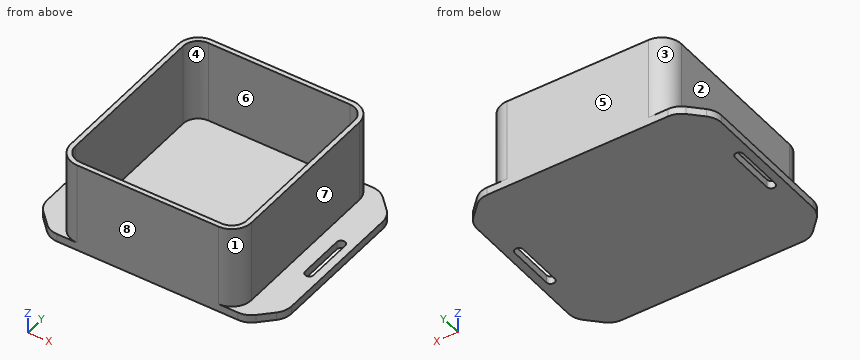
```python
from build123d import *

# Parameters (mm, degrees)
F1_DEPTH = 2
F3_DEPTH = 21


with BuildPart() as f1:
    # F0 (on Top) → F1 (new body)
    with BuildSketch(Plane.XY):
        with BuildLine():
            Line((-60.535534, 4.535534), (-57.464466, 1.464466))
            ThreePointArc((-57.464466, 1.464466), (-55.842349, 0.380602), (-53.928932, 0))
            Line((-53.928932, 0), (-8.071068, 0))
            ThreePointArc((-8.071068, 0), (-6.157651, 0.380602), (-4.535534, 1.464466))
            Line((-4.535534, 1.464466), (-1.464466, 4.535534))
            ThreePointArc((-1.464466, 4.535534), (-0.380602, 6.157651), (0, 8.071068))
            Line((0, 8.071068), (0, 41.928932))
            ThreePointArc((0, 41.928932), (-0.380602, 43.842349), (-1.464466, 45.464466))
            Line((-1.464466, 45.464466), (-4.535534, 48.535534))
            ThreePointArc((-4.535534, 48.535534), (-6.157651, 49.619398), (-8.071068, 50))
            Line((-8.071068, 50), (-53.928932, 50))
            ThreePointArc((-53.928932, 50), (-55.842349, 49.619398), (-57.464466, 48.535534))
            Line((-57.464466, 48.535534), (-60.535534, 45.464466))
            ThreePointArc((-60.535534, 45.464466), (-61.619398, 43.842349), (-62, 41.928932))
            Line((-62, 41.928932), (-62, 8.071068))
            ThreePointArc((-62, 8.071068), (-61.619398, 6.157651), (-60.535534, 4.535534))
        make_face()
        with BuildLine():
            Line((-60, 19.118238), (-60, 30.881762))
            ThreePointArc((-60, 30.881762), (-58.930589, 31.951173), (-57.861177, 30.881762))
            Line((-57.861177, 30.881762), (-57.861177, 19.118238))
            ThreePointArc((-57.861177, 19.118238), (-58.930589, 18.048827), (-60, 19.118238))
        make_face(mode=Mode.SUBTRACT)
        with BuildLine():
            Line((-4.138823, 19.118238), (-4.138823, 30.881762))
            ThreePointArc((-4.138823, 30.881762), (-3.069411, 31.951173), (-2, 30.881762))
            Line((-2, 30.881762), (-2, 19.118238))
            ThreePointArc((-2, 19.118238), (-3.069411, 18.048827), (-4.138823, 19.118238))
        make_face(mode=Mode.SUBTRACT)
    extrude(amount=F1_DEPTH)

    # F2 (on face) → F3 (join)
    with BuildSketch(Plane.XY.offset(2)):
        with BuildLine():
            ThreePointArc((-13.071068, 0), (-9.535534, 1.464466), (-8.071068, 5))
            Line((-8.071068, 5), (-8.071068, 45))
            ThreePointArc((-8.071068, 45), (-9.535534, 48.535534), (-13.071068, 50))
            Line((-13.071068, 50), (-48.928932, 50))
            ThreePointArc((-48.928932, 50), (-52.464466, 48.535534), (-53.928932, 45))
            Line((-53.928932, 45), (-53.928932, 5))
            ThreePointArc((-53.928932, 5), (-52.464466, 1.464466), (-48.928932, 0))
            Line((-48.928932, 0), (-13.071068, 0))
        make_face()
        with BuildLine():
            Line((-9.271068, 45), (-9.271068, 5))
            ThreePointArc((-9.271068, 5), (-10.384062, 2.312995), (-13.071068, 1.200001))
            Line((-13.071068, 1.200001), (-48.928932, 1.200001))
            ThreePointArc((-48.928932, 1.200001), (-51.615938, 2.312995), (-52.728932, 5))
            Line((-52.728932, 5), (-52.728932, 45))
            ThreePointArc((-52.728932, 45), (-51.615938, 47.687005), (-48.928932, 48.799999))
            Line((-48.928932, 48.799999), (-13.071068, 48.799999))
            ThreePointArc((-13.071068, 48.799999), (-10.384062, 47.687005), (-9.271068, 45))
        make_face(mode=Mode.SUBTRACT)
    extrude(amount=F3_DEPTH)


solid = f1.part
```
Read the model definition and answer for the solid it produces. Units are mm, in the model's axes. Face numbers are marked on the shaded views. A direction names the side the tool comes from. Give positions to 0.01 mm unless a question says otherwise; leave off trailing zeros. Order: outer loops, then holes, each group sorted by start corner. A loop starts at its lowest first (then second) coordinate and runs counter-clockwise, first axis right, second up. Notation, with made-up numbers: (74.5, -14.5) -> (131.5, -14.5) arc R17 cw to (131.5, 12.5) -> close; hole circle Ø8 at (-6.75, 10.25). An arc over 180 degrees is marked (long way). One line per item, written item: value. Start each with the question number.
(1) Straight lines are drawn through the part: L1, parallel to X at y = 7, z = 20; L2, parallel to Y at x = -24, z = 7.25; L3, parallel to Z at x = -11.5, y = 25. For each, find the intervals that lie inside material, in ascending order.
(2) The part is cut by section B-B (z = 16.5). Determine the outline of the cut face in (x, y), and give its area (3 significant figures).
(3) A tool of negligible diameter and unlimited length cuts with its end or side. For the marked faces 1, 2, 3, 4 and 5, from which of +Z, -Z, +X, -X, +Y, -Y can it reach the whole face along a straight path? Write none if from no direction.
(4) The part is cut by section C-C (x = -50.5). Determine the outline of the cut face in (y, z), and give its area (3 significant figures).
(5) Flat-ended cylindrical pins translate along their axes: P1, Ø6.5, axis at y = 29.5, z = 10, coming from the +X side; P2, Ø10, axis at y = 44.5, z = 15.5, coming from the -X side; P3, Ø4, axis at x = -4.5, y = 33, coming from the +Z side. Find the tip coordinate at first contact, or state that the pin passes through.
(6) For a pull along X with two mould halves and no side action, classify the marked faces 6, 7 and 8 as released by +X, released by -X, zero draft, split by the parting line, or undercut.
(7) The part is cut by section D-D (y = 47.5). Determine the outline of the cut face in (x, z).
(8) The part is cut by section A-A (y = 29). Determine the outline of the cut face in (x, z).
Taken from the geometry:
1. L1: -53.93 to -52.73, -9.27 to -8.07
1. L2: 0 to 1.2, 48.8 to 50
1. L3: 0 to 2
2. outline: (-53.93, 5) arc R5 ccw to (-48.93, 0) -> (-13.07, 0) arc R5 ccw to (-8.07, 5) -> (-8.07, 45) arc R5 ccw to (-13.07, 50) -> (-48.93, 50) arc R5 ccw to (-53.93, 45) -> close; hole (-52.73, 5) arc R3.8 ccw to (-48.93, 1.2) -> (-13.07, 1.2) arc R3.8 ccw to (-9.27, 5) -> (-9.27, 45) arc R3.8 ccw to (-13.07, 48.8) -> (-48.93, 48.8) arc R3.8 ccw to (-52.73, 45) -> close
2. area: 215 mm^2
3. face 1: +Z, +X, -Y
3. face 2: +Z, -X, +Y, -Y
3. face 3: +Z, -X, +Y
3. face 4: +Z
3. face 5: +Z, -Z, +X, -X, +Y
4. outline: (0, 0) -> (50, 0) -> (50, 2) -> (49.75, 2) -> (49.75, 23) -> (48.46, 23) -> (48.46, 2) -> (1.54, 2) -> (1.54, 23) -> (0.25, 23) -> (0.25, 2) -> (0, 2) -> close
4. area: 154 mm^2
5. P1: x = -8.07
5. P2: x = -53.93
5. P3: z = 2
6. face 6: undercut
6. face 7: released by +X
6. face 8: zero draft
7. outline: (-58.5, 0) -> (-3.5, 0) -> (-3.5, 2) -> (-8.74, 2) -> (-8.74, 23) -> (-10.21, 23) -> (-10.21, 2) -> (-51.79, 2) -> (-51.79, 23) -> (-53.26, 23) -> (-53.26, 2) -> (-58.5, 2) -> close
8. outline: (-62, 0) -> (-60, 0) -> (-60, 2) -> (-62, 2) -> close; (-57.86, 0) -> (-4.14, 0) -> (-4.14, 2) -> (-8.07, 2) -> (-8.07, 23) -> (-9.27, 23) -> (-9.27, 2) -> (-52.73, 2) -> (-52.73, 23) -> (-53.93, 23) -> (-53.93, 2) -> (-57.86, 2) -> close; (-2, 0) -> (0, 0) -> (0, 2) -> (-2, 2) -> close
